from build123d import *

# Parameters (mm, degrees)
SKETCH1_R           = 15
BOSS_EXTRUDE1_DEPTH = 60
BOSS_EXTRUDE2_DEPTH = 15
SKETCH3_R           = 5
BOSS_EXTRUDE3_DEPTH = 15
SKETCH4_R           = 5
CUT_EXTRUDE1_DEPTH  = 146


with BuildPart() as part:
    # Sketch1 → Boss-Extrude1 (new body)
    with BuildSketch(Plane.XY):
        Circle(SKETCH1_R)
    extrude(amount=BOSS_EXTRUDE1_DEPTH)

    # Sketch2 → Boss-Extrude2 (add, symmetric)
    with BuildSketch(Plane(origin=(0, 0, 0), x_dir=(1, 0, 0), z_dir=(0, 1, 0))):
        Polygon((0, 0), (-20, 0), (-20, -30), (-17, -30), (-17, -3), (0, -3), align=None)
    boss_extrude2 = extrude(amount=BOSS_EXTRUDE2_DEPTH, both=True)

    # Mirror1: Boss-Extrude2 across plane
    add(boss_extrude2.mirror(Plane(origin=(-17, -15, 30), x_dir=(1, 0, 0), z_dir=(0, 0, 1))))

    # Sketch3 → Boss-Extrude3 (add)
    with BuildSketch(Plane.ZY.offset(20)):
        with Locations((30, 0)):
            Circle(SKETCH3_R)
    extrude(amount=BOSS_EXTRUDE3_DEPTH)

    # Sketch4 → Cut-Extrude1 (cut)
    with BuildSketch(Plane.XY.offset(60)):
        Circle(SKETCH4_R)
    extrude(amount=-CUT_EXTRUDE1_DEPTH, mode=Mode.SUBTRACT)


solid = part.part
Here's how the part is built. I have some questions about the finished solid (model axes, mm). A direction names the side the tool comes from. Round coordinates to 2 decimals unless told otherwise and drop trailing zeros. Loops run counter-clockwise (first coordinate to the right, second up) from the corner with the lowest first, then second, coordinate; pieces in that order, holes last. Notation, with made-up numbers: (24.5, 30.5) - (39.5, 30.5) arc R23 ccw to (39.5, 41.5) - close; hole circle Ø7 at (-25, -22.75). An arc over 180 degrees is marked (long way). One line per question, with ' | ' between items. Start each with the question number.
Q1. Please list where these lines run through material, in increasing order: line 1 (Y direction, x = 0, z = 31); line 2 (Z direction, x = -9, y = -13); line 3 (X direction, y = -2.75, z = 45). Write a range as [from, to].
Q2. Will these pins go through, and if not, where does the flat tip stop? pin 1 (8 mm diameter, centred on y = 5.5, z = 44, fed in from -X); pin 2 (10 mm diameter, centred on x = -5.5, z = 51.5, fed in from +Y); pin 3 (4 mm diameter, centred on x = 2.5, z = 37, fed in from -Y).
Q3. We'd pull the mould along X, two halves only. Please class faces 1 (the flat face through (-6, 0, 0)), 2 (the flat face through (-35, 0, 30)), 3 (the cylindrical face through (-1.08, -4.88, 30.42)), 4 (the cylindrical face through (13.856, -5.745, 29.58)): +X half, -X half, draft (parallel to the pull), parting line (faces both ways), or undercut.
Q4. I want a section at B-B (z = 30). Write out the boundary of the cut face in (x, y), then the cut area to 3 significant figures.
Q5. For faces 5 (the flat face through (-17, 0, 30)), 6 (the cylindrical face through (-27, 0, 25)), 7 (the flat face through (-15.5, 0.1, 57)), which set-ups out of +Z, -Z, +X, -X, +Y, -Y let a thin tool reach every point of the face, with its end or its side?
Q6. I want a section at C-C (z = 9). Write out the boundary of the cut face in (x, y), then the cut area to 3 significant figures.
Q7. I want a section at A-A (y = 0). Write out the boundary of the cut face in (x, z), then the cut area to 3 significant figures.
Q8. I want a section at D-D (y = 6.5). Write out the boundary of the cut face in (x, z).
Response values:
1) line 1: y = [-15, -5], [5, 15] | line 2: z = [0, 3], [57, 60] | line 3: x = [-20, -17], [-14.75, -4.18], [4.18, 14.75]
2) pin 1: stops at x = -20 | pin 2: stops at y = 14.99 | pin 3: stops at y = -14.99
3) face 1: draft | face 2: -X half | face 3: undercut | face 4: undercut
4) outline: (-35, -5) - (-20, -5) - (-20, -15) - (-17, -15) - (-17, 15) - (-20, 15) - (-20, 5) - (-35, 5) - close; circle Ø30 at (0, 0); hole circle Ø10 at (0, 0) | area: 868 mm²
5) face 5: +Y, -Y | face 6: -X | face 7: none
6) outline: (-20, -15) - (-17, -15) - (-17, 15) - (-20, 15) - close; circle Ø30 at (0, 0); hole circle Ø10 at (0, 0) | area: 718 mm²
7) outline: (-35, 25) - (-20, 25) - (-20, 0) - (-5, 0) - (-5, 60) - (-20, 60) - (-20, 35) - (-35, 35) - close; (5, 0) - (15, 0) - (15, 60) - (5, 60) - close; hole (-17, 3) - (-15, 3) - (-15, 57) - (-17, 57) - close | area: 1,540 mm²
8) outline: (-20, 0) - (13.52, 0) - (13.52, 60) - (-20, 60) - close; hole (-17, 3) - (-13.52, 3) - (-13.52, 57) - (-17, 57) - close
